from build123d import *

# Parameters (mm, degrees)
SKETCH1_W           = 50
SKETCH1_H           = 25
BOSS_EXTRUDE1_DEPTH = 250
SHELL1_T            = -3
SKETCH2_W           = 50
SKETCH2_H           = 25
BOSS_EXTRUDE2_DEPTH = 110
SKETCH3_W           = 28.35
SKETCH3_H           = 31.35
CUT_EXTRUDE1_DEPTH  = 107
SKETCH4_W           = 28.35
SKETCH4_H           = 5
CUT_EXTRUDE2_DEPTH  = 3
SKETCH5_R           = 1.45
CUT_EXTRUDE3_DEPTH  = 10
SKETCH6_W           = 8
SKETCH6_H           = 2
CUT_EXTRUDE4_DEPTH  = 10
SKETCH7_W           = 22.35
SKETCH7_H           = 23.35
CUT_EXTRUDE5_DEPTH  = 10
SKETCH9_W           = 110
SKETCH9_H           = 50
BOSS_EXTRUDE3_DEPTH = 3
SKETCH10_R          = 15.2
CUT_EXTRUDE6_DEPTH  = 3
SKETCH11_R          = 3
BOSS_EXTRUDE4_DEPTH = 15
SKETCH12_R          = 1.45
CUT_EXTRUDE7_DEPTH  = 10
SKETCH13_R          = 1.6
CUT_EXTRUDE8_DEPTH  = 10
CHAMFER1_SIZE       = 1


with BuildPart() as part:
    # Sketch1 → Boss-Extrude1 (new body)
    with BuildSketch(Plane(origin=(0, 0, 0), x_dir=(0, 0, -1), z_dir=(1, 0, 0))):
        with BuildLine():
            ThreePointArc((23.062381853, -6.238185255), (20.988557625, -14.697361116), (15.237381853, -21.238185255))
            Line((15.237381853, -21.238185255), (-19.112618147, -21.238185255))
            ThreePointArc((-19.112618147, -21.238185255), (-24.86379392, -14.697361116), (-26.937618147, -6.238185255))
            Line((-26.937618147, -6.238185255), (23.062381853, -6.238185255))
        make_face()
        with Locations((-1.937618147, 6.261814745)):
            Rectangle(SKETCH1_W, SKETCH1_H)
    extrude(amount=BOSS_EXTRUDE1_DEPTH)

    # Shell1
    shell1_openings = [part.faces().sort_by_distance(p)[0] for p in [
        (125, 18.761814745, 1.937618147),
    ]]
    offset(amount=SHELL1_T, openings=shell1_openings, kind=Kind.INTERSECTION)

    # Sketch2 → Boss-Extrude2 (add)
    with BuildSketch(Plane.ZY):
        with Locations((1.937618147, 6.261814745)):
            Rectangle(SKETCH2_W, SKETCH2_H)
        with BuildLine():
            Line((-23.062381853, -6.238185255), (26.937618147, -6.238185255))
            ThreePointArc((26.937618147, -6.238185255), (24.86379392, -14.697361116), (19.112618147, -21.238185255))
            Line((19.112618147, -21.238185255), (-15.237381853, -21.238185255))
            ThreePointArc((-15.237381853, -21.238185255), (-20.988557625, -14.697361116), (-23.062381853, -6.238185255))
        make_face()
    extrude(amount=-BOSS_EXTRUDE2_DEPTH)

    # Sketch3 → Cut-Extrude1 (cut)
    with BuildSketch(Plane.ZY):
        with Locations((1.937618147, -5.563185255)):
            Rectangle(SKETCH3_W, SKETCH3_H)
    extrude(amount=-CUT_EXTRUDE1_DEPTH, mode=Mode.SUBTRACT)

    # Sketch4 → Cut-Extrude2 (cut)
    with BuildSketch(Plane.ZY):
        with Locations((1.937618147, 12.611814745)):
            Rectangle(SKETCH4_W, SKETCH4_H)
    extrude(amount=-CUT_EXTRUDE2_DEPTH, mode=Mode.SUBTRACT)

    # Sketch5 → Cut-Extrude3 (cut)
    with BuildSketch(Plane.ZY.offset(-3)):
        with Locations((-7.062381853, 12.611814745)):
            Circle(SKETCH5_R)
        with Locations((10.937618147, 12.611814745)):
            Circle(SKETCH5_R)
    extrude(amount=-CUT_EXTRUDE3_DEPTH, mode=Mode.SUBTRACT)

    # Sketch6 → Cut-Extrude4 (cut)
    with BuildSketch(Plane.ZY.offset(-107)):
        with Locations((1.937618147, -19.238185255)):
            Rectangle(SKETCH6_W, SKETCH6_H)
    extrude(amount=-CUT_EXTRUDE4_DEPTH, mode=Mode.SUBTRACT)

    # Sketch7 → Cut-Extrude5 (cut)
    with BuildSketch(Plane.ZY.offset(-107)):
        with Locations((1.937618147, -4.563185255)):
            Rectangle(SKETCH7_W, SKETCH7_H)
    extrude(amount=-CUT_EXTRUDE5_DEPTH, mode=Mode.SUBTRACT)

    # Sketch9 → Boss-Extrude3 (add)
    with BuildSketch(Plane(origin=(0, 18.761814745, 0), x_dir=(1, 0, 0), z_dir=(0, 1, 0))):
        with Locations((55, -1.937618147)):
            Rectangle(SKETCH9_W, SKETCH9_H)
    extrude(amount=BOSS_EXTRUDE3_DEPTH)

    # Sketch10 → Cut-Extrude6 (cut)
    with BuildSketch(Plane(origin=(250, 0, 0), x_dir=(0, 0, -1), z_dir=(1, 0, 0))):
        with Locations((-1.937618147, -1.238185255)):
            Circle(SKETCH10_R)
    extrude(amount=-CUT_EXTRUDE6_DEPTH, mode=Mode.SUBTRACT)

    # Sketch11 → Boss-Extrude4 (add)
    with BuildSketch(Plane(origin=(0, 18.761814745, 0), x_dir=(1, 0, 0), z_dir=(0, 1, 0))):
        with Locations((247, -23.937618147)):
            Circle(SKETCH11_R)
        with Locations((247, 20.062381853)):
            Circle(SKETCH11_R)
        with Locations((113, 20.062381853)):
            Circle(SKETCH11_R)
        with Locations((113, -23.937618147)):
            Circle(SKETCH11_R)
    extrude(amount=-BOSS_EXTRUDE4_DEPTH)

    # Sketch12 → Cut-Extrude7 (cut)
    with BuildSketch(Plane(origin=(0, 18.761814745, 0), x_dir=(1, 0, 0), z_dir=(0, 1, 0))):
        with Locations(Location((113, 20.062381853, 0), (0, 0, 270))):
            Circle(SKETCH12_R)
        with Locations(Location((113, -23.937618147, 0), (0, 0, 270))):
            Circle(SKETCH12_R)
        with Locations(Location((247, -23.937618147, 0), (0, 0, 270))):
            Circle(SKETCH12_R)
        with Locations(Location((247, 20.062381853, 0), (0, 0, 270))):
            Circle(SKETCH12_R)
    extrude(amount=-CUT_EXTRUDE7_DEPTH, mode=Mode.SUBTRACT)

    # Sketch13 → Cut-Extrude8 (cut)
    with BuildSketch(Plane(origin=(0, -18.238185255, 0), x_dir=(1, 0, 0), z_dir=(0, 1, 0))):
        with Locations(Location((150, 10.063881853, 0), (0, 0, 270))):
            Circle(SKETCH13_R)
        with Locations(Location((150, -13.939118147, 0), (0, 0, 270))):
            Circle(SKETCH13_R)
        with Locations(Location((196.482, -13.939118147, 0), (0, 0, 270))):
            Circle(SKETCH13_R)
        with Locations(Location((196.482, 10.063881853, 0), (0, 0, 270))):
            Circle(SKETCH13_R)
    extrude(amount=-CUT_EXTRUDE8_DEPTH, mode=Mode.SUBTRACT)

    # Chamfer1
    chamfer1_edges = [part.edges().sort_by_distance(p)[0] for p in [
        (196.482, -21.238185255, -11.663881853),
        (196.482, -21.238185255, 12.339118147),
        (150, -21.238185255, 12.339118147),
        (150, -21.238185255, -11.663881853),
    ]]
    chamfer(chamfer1_edges, length=CHAMFER1_SIZE)


solid = part.part
Can you work these out from the model? Positions are in its coordinate system, mm. A direction names the side the tool comes from. Give positions to 0.01 mm unless a question says otherwise; leave off trailing zeros. Order: outer loops, then holes, each group sorted by start corner. A loop starts at its lowest first (then second) coordinate and runs counter-clockwise, first axis right, second up. Notation, with made-up numbers: (27, -33) - (84, -33) arc R20 cw to (84, -22) - close; hole circle Ø7 at (20.25, 81). An arc over 180 degrees is marked (long way). Write each question's results on one line, items separated by ' | '.
1) If we mould it in two halves opening along Z, with no side actions, what happens to faces 1 (the face through (123.25, -14.806, 24.806)), 2 (the face through (0, 19, 2)), 3 (the face through (112.934, 11.367, -17.063))? For each: pulls with the +Z half, pulls with the -Z half, needs draft (parallel to the pull), parting line crosses it, or undercut.
Final values:
face 1: pulls with the +Z half | face 2: needs draft | face 3: undercut
2) Suppose I cut it at A-A, the plane z = 0.5. Write out the boundary of the cut face in (x, y), then the cut area to 3 significant figures.
Final values:
outline: (0, 15.11) - (3, 15.11) - (3, 10.11) - (107, 10.11) - (107, 7.11) - (110, 7.11) - (110, 21.76) - (0, 21.76) - close; (107, -21.24) - (250, -21.24) - (250, -16.37) - (247, -16.37) - (247, -18.24) - (117, -18.24) - (117, -20.24) - (107, -20.24) - close; (107, -18.24) - (110, -18.24) - (110, -16.24) - (107, -16.24) - close; (247, 13.89) - (250, 13.89) - (250, 18.76) - (247, 18.76) - close | area: 1,710 mm^2
3) Suppose I cut it at B-B, the plane x = 233.5. Write out the boundary of the cut face in (y, z), then the cut area to 3 significant figures.
Final values:
outline: (-21.24, -15.24) arc R18.29 ccw to (-6.24, -23.06) - (18.76, -23.06) - (18.76, -20.06) - (-6.24, -20.06) arc R15.29 cw to (-18.24, -14.25) - (-18.24, 18.12) arc R15.29 cw to (-6.24, 23.94) - (18.76, 23.94) - (18.76, 26.94) - (-6.24, 26.94) arc R18.29 ccw to (-21.24, 19.11) - close | area: 344 mm^2
4) Suppose I cut it at C-C, the plane x = 104. Write out the boundary of the cut face in (y, z), then the cut area to 3 significant figures.
Final values:
outline: (-21.24, -15.24) arc R18.29 ccw to (-6.24, -23.06) - (21.76, -23.06) - (21.76, 26.94) - (-6.24, 26.94) arc R18.29 ccw to (-21.24, 19.11) - (-21.24, 16.11) - (10.11, 16.11) - (10.11, -12.24) - (-21.24, -12.24) - close | area: 1,190 mm^2
5) On a 3-axis mill with a long thin cutter (end or side, diameter ignored), from which of +Z, -Z, +X, -X, +Y, -Y can I reach the whole of each face in a straight line? I mean faces 4 (the face through (112, -20.238, 2)), 5 (the face through (151, -21.238, 2)), 6 (the face through (190, 18.762, 24.3)), 7 (the face through (54, 10.112, 2)), 8 (the face through (178, -18.238, 2)). Say none if no direction works.
Final values:
face 4: -X | face 5: +Z, -Z, +X, -X, -Y | face 6: +Z, -Z, +X, +Y | face 7: -X, -Y | face 8: +Y
6) Please list where these lines run through material, in increasing order: line 1 along Z through (x, y) = (100, 8.5); line 2 along Z through (x, y) = (86, -7.5); line 3 along Z through (x, y) = (113, 14.5). Write a range as [from, to].
Final values:
line 1: z = [-23.06, -12.24], [16.11, 26.94] | line 2: z = [-23.02, -12.24], [16.11, 26.89] | line 3: z = [-23.06, -21.51], [-18.61, -17.06], [20.94, 22.49], [25.39, 26.94]
7) I'm going to push flat-ended pins straight in: pin 1 Ø0.9 at (x, z) = (112.5, -19.5) entering from +Y; pin 2 Ø1.5 at (y, z) = (-6.5, 11.5) entering from +X; pin 3 Ø0.9 at (x, z) = (114, -18.5) entering from -Y; pin 4 Ø2.5 at (x, z) = (245, 22.5) entering from -Y. Where does each tip first touch, or does it pass through?
Final values:
pin 1: stops at y = 8.76 | pin 2: passes through | pin 3: stops at y = -18.82 | pin 4: stops at y = -19.49
